from build123d import *

# Parameters (mm, degrees)
EXTRUDE_1_DEPTH      = 2
EXTRUDE_2_DEPTH      = 10
EXTRUDE_2_DEPTH_BACK = 10
SKETCH_3_R           = 1.5
CUT_EXTRUDE_1_DEPTH  = 103.571925984
SKETCH_4_R           = 1.5
CUT_EXTRUDE_2_DEPTH  = 103.571925984
FILLET_1_R           = 1


with BuildPart() as part:
    # 草图1 → 凸台-拉伸1 (new body)
    with BuildSketch(Plane(origin=(0, 0, 0), x_dir=(1, 0, 0), z_dir=(0, 1, 0))):
        Polygon((0, 100), (0, 0), (20, 0), align=None)
    extrude(amount=EXTRUDE_1_DEPTH)

    # 草图2 → 凸台-拉伸2 (add, two sides: drawn at the far end of the back side and taken through both)
    with BuildSketch(Plane(origin=(0, 1, 0), x_dir=(-1, 0, 0), z_dir=(0, -1, 0)).offset(-EXTRUDE_2_DEPTH_BACK)):
        Polygon((-20, 0), (-20, -3), (3, -3), (3, 100), (0, 100), (0, 0), align=None)
    extrude(amount=EXTRUDE_2_DEPTH + EXTRUDE_2_DEPTH_BACK)

    # 草图3 → 切除-拉伸1 (cut, through all)
    with BuildSketch(Plane(origin=(0, 0, 0), x_dir=(0, 0, -1), z_dir=(1, 0, 0))):
        with Locations((95, 6.5)):
            Circle(SKETCH_3_R)
        with Locations((35, 6.5)):
            Circle(SKETCH_3_R)
        with Locations(Location((95, -4.5, 0), (0, 0, 180))):
            Circle(SKETCH_3_R)
        with Locations(Location((35, -4.5, 0), (0, 0, 180))):
            Circle(SKETCH_3_R)
    extrude(amount=-CUT_EXTRUDE_1_DEPTH, mode=Mode.SUBTRACT)

    # 草图4 → 切除-拉伸2 (cut, through all)
    with BuildSketch(Plane(origin=(0, 0, 0), x_dir=(-1, 0, 0), z_dir=(0, 0, -1))):
        with Locations((-17, 8)):
            Circle(SKETCH_4_R)
        with Locations(Location((-17, -6, 0), (0, 0, 180))):
            Circle(SKETCH_4_R)
        with Locations((-3, -6)):
            Circle(SKETCH_4_R)
        with Locations(Location((-3, 8, 0), (0, 0, 180))):
            Circle(SKETCH_4_R)
    extrude(amount=-CUT_EXTRUDE_2_DEPTH, mode=Mode.SUBTRACT)

    # 圆角1
    fillet_1_edges = [part.edges().sort_by_distance(p)[0] for p in [
        (10, 2, 0),
        (10, 0, 0),
    ]]
    fillet(fillet_1_edges, radius=FILLET_1_R)


solid = part.part
Check sheet for the modelled part. Datum: model origin and axes. Units: mm. A direction names the side the tool comes from. Round coordinates to 2 decimals unless told otherwise and drop trailing zeros. Loops run counter-clockwise (first coordinate to the right, second up) from the corner with the lowest first, then second, coordinate; pieces in that order, holes last. Notation, with made-up numbers: (-3.5, 89) - (4.5, 89) arc R19 cw to (4.5, 111) - close; hole circle Ø11 at (85, 57.5). An arc over 180 degrees is marked (long way). Answer as CSV lines item,"result". Start each with the question number.
Item 1: Scan lines: line 1 (Y direction, x = 3, z = 0.9); line 2 (Z direction, x = -2.25, y = -4.5); line 3 (Y direction, x = -1.2, z = -35). Record each from-to range of solid material in increasing order. Write a range as [from, to].
Item 2: Section check A-A (z = -35). Record the boundary of the cut face in (x, y).
Item 3: Section check C-C (z = -9.5). Record the boundary of the cut face in (x, y).
Item 4: Section check B-B (x = 17). Record the boundary of the cut face in (y, z), and give its area (3 significant figures).
Item 5: Set-up check for faces 1 (the cylindrical face through (1.57, -5.55, 1.48)), 2 (the flat face through (5, 0, -29)), 3 (the flat face through (0, 7, -51)): record each of +Z, -Z, +X, -X, +Y, -Y from which the full face is reachable in a straight line by a thin tool's end or side.
Item 6: Depth check by flat-ended pin: P1, Ø10, axis at x = 8, z = -74, coming from the +Y side; P2, Ø6, axis at x = 10, z = -72, coming from the -Y side; P3, Ø10, axis at y = -6, z = -55.5, coming from the +X side; P4, Ø6.5, axis at x = 12, y = -4, coming from the -Z side. Enter the tip coordinate at first touch or a pass-through.
Item 7: Release check for a two-part mould opening along Z. For faces 4 (the flat face through (10, -5, 0)), 5 (the cylindrical face through (-1.5, 5.6, -33.8)), 6 (the cylindrical face through (18.5, 8.07, 1.48)) record: +Z half, -Z half, draft (parallel to the pull), parting line (faces both ways), or undercut.
Item 8: Section check D-D (x = 3). Record the boundary of the cut face in (y, z), and give its area (3 significant figures).
Report:
1,line 1,"y = [-9, -7.5], [-4.5, 6.5], [9.5, 11]"
1,line 2,"z = [-100, -96.5], [-93.5, -36.5], [-33.5, 3]"
1,line 3,"y = [-9, -6], [-3, 5], [8, 11]"
2,outline,"(-3, -9) - (0, -9) - (0, -6) - (-3, -6) - close; (-3, -3) - (0, -3) - (0, 0) - (13, 0) - (13, 2) - (0, 2) - (0, 5) - (-3, 5) - close; (-3, 8) - (0, 8) - (0, 11) - (-3, 11) - close"
3,outline,"(-3, -9) - (0, -9) - (0, 0) - (18.1, 0) - (18.1, 2) - (0, 2) - (0, 11) - (-3, 11) - close"
4,outline,"(-9, 0) - (-7.5, 0) - (-7.5, 3) - (-9, 3) - close; (-4.5, 0) - (-1, 0) arc R1 cw to (0, -1) - (0, -15) - (2, -15) - (2, -1) arc R1 cw to (3, 0) - (6.5, 0) - (6.5, 3) - (-4.5, 3) - close; (9.5, 0) - (11, 0) - (11, 3) - (9.5, 3) - close"
4,area,"72.4 mm2"
5,face 1,"+Z, -Z"
5,face 2,"-Z, +X, -Y"
5,face 3,"-Z, +X, +Y"
6,P1,"stops at y = 2"
6,P2,"passes through"
6,P3,"stops at x = 0"
6,P4,"stops at z = -0.03"
7,face 4,"-Z half"
7,face 5,"undercut"
7,face 6,"draft"
8,outline,"(-9, 0) - (-7.5, 0) - (-7.5, 3) - (-9, 3) - close; (-4.5, 0) - (-1, 0) arc R1 cw to (0, -1) - (0, -85) - (2, -85) - (2, -1) arc R1 cw to (3, 0) - (6.5, 0) - (6.5, 3) - (-4.5, 3) - close; (9.5, 0) - (11, 0) - (11, 3) - (9.5, 3) - close"
8,area,"212 mm2"
